Here's how the part is built. I have some questions about the finished solid (model axes, mm). Face numbers are marked on the shaded views. A direction names the side the tool comes from. Coordinates: 2 decimals unless noted, no trailing zeros. Write each loop counter-clockwise with the first axis right and the second up, starting at its lowest first coordinate (ties: lowest second). Pieces come first, ordered by that corner, then holes.
Item 1: If we section it at A-A (y = 0): Please give me the cut outline in (x, z).
Item 2: If we section it at C-C (y = -3): Please give me the cut outline in (x, z), then the cut area to 3 significant figures.
Item 3: I'm going to push flat-ended pins straight in: pin 1 Ø2 at (x, z) = (3, 0) entering from +Y; pin 2 Ø1.5 at (x, z) = (1.5, 1.5) entering from -Y; pin 3 Ø1.5 at (y, z) = (-3, -0.5) entering from -X. Where does each tip first touch, or does it pass through?
Item 4: We'd pull the mould along X, two halves only. Please class the marked faces 3, 4 and 5: +X half, -X half, draft (parallel to the pull), parting line (faces both ways), or undercut.
Item 5: For the marked faces 1 and 2, which set-ups out of +Z, -Z, +X, -X, +Y, -Y let a thin tool reach every point of the face, with its end or its side?
Item 6: If we section it at D-D (z = -0.35): Please give me the cut outline in (x, y), then the cut area to 3 significant figures.
Item 7: If I drill on line 1 (Y direction, x = 0, z = -0.8); line 2 (Z direction, x = -3, y = 1); line 3 (Y direction, x = -1.25, z = 1.45), over which ranges is the centre line in solid material (lowest first)?
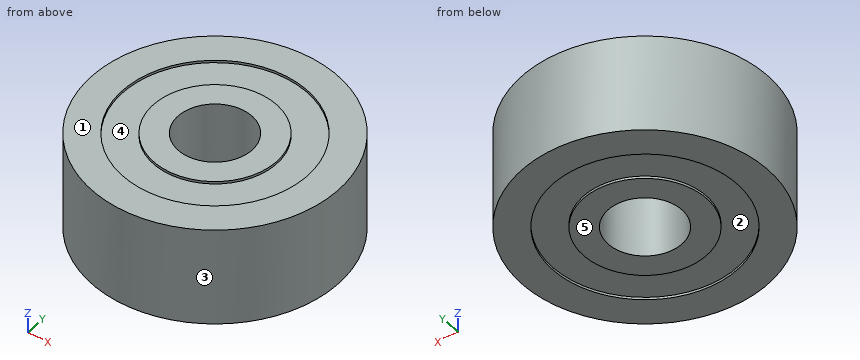
Autodesk Inventor part; units mm, degrees
ref_plane "YZ Plane" through (0, 0, 0) normal (1, 0, 0) x (0, 1, 0)
ref_plane "XZ Plane" through (0, 0, 0) normal (0, 1, 0) x (-1, 0, 0)
ref_plane "XY Plane" through (0, 0, 0) normal (0, 0, 1) x (1, 0, 0)
sketch "Sketch1" plane through (0, 0, 0) normal (0, 0, 1) x (1, 0, 0)
  circle A0 centre (0, 0) radius 1.5
  circle A1 centre (0, 0) radius 5
  dimension "d0" = 3
  dimension "d1" = 10
extrude "Extrusion1" add sketch "Sketch1" along normal mid plane 4
sketch "Sketch2" plane through (0, 0, 2) normal (0, 0, 1) x (1, 0, 0)
  circle A0 centre (0, 0) radius 1.5
  circle A1 centre (0, 0) radius 5
  circle A2 centre (0, 0) radius 3.75
  circle A3 centre (0, 0) radius 2.5
  dimension "d4" = 1.25
  dimension "d5" = 1
extrude "Extrusion2" cut sketch "Sketch2" against normal blind 0.1 contours A2
mirror "Mirror1" about plane through (0, 0, 0) normal (0, 0, 1) of "Extrusion2"
properties part number "idler bearing"
Answer list:
1. outline: (-5, -2) - (-3.75, -2) - (-3.75, -1.9) - (-2.5, -1.9) - (-2.5, -2) - (-1.5, -2) - (-1.5, 2) - (-2.5, 2) - (-2.5, 1.9) - (-3.75, 1.9) - (-3.75, 2) - (-5, 2) - close; (1.5, -2) - (2.5, -2) - (2.5, -1.9) - (3.75, -1.9) - (3.75, -2) - (5, -2) - (5, 2) - (3.75, 2) - (3.75, 1.9) - (2.5, 1.9) - (2.5, 2) - (1.5, 2) - close
2. outline: (-4, -2) - (-2.25, -2) - (-2.25, -1.9) - (2.25, -1.9) - (2.25, -2) - (4, -2) - (4, 2) - (2.25, 2) - (2.25, 1.9) - (-2.25, 1.9) - (-2.25, 2) - (-4, 2) - close
2. area: 31.1 mm2
3. pin 1: stops at y = 4.58
3. pin 2: stops at y = -4.94
3. pin 3: stops at x = -4.47
4. face 3: parting line
4. face 4: undercut
4. face 5: draft
5. face 1: +Z, +X, -X, +Y, -Y
5. face 2: -Z
6. outline: circle Ø10 at (0, 0); hole circle Ø3 at (0, 0)
6. area: 71.5 mm2
7. line 1: y = -5 to -1.5, 1.5 to 5
7. line 2: z = -1.9 to 1.9
7. line 3: y = -4.84 to -0.83, 0.83 to 4.84
